```python
from build123d import *

# Parameters (mm, degrees)
RECESSII_CUT_EXTRUDE11_DEPTH = 2.0574
DRAFT2_ANGLE                 = 20
LPATTERN1_COUNT              = 9
LPATTERN1_PITCH              = 1.27


with BuildPart() as part:
    # Sketch1 → base-Revolve (revolve)
    with BuildSketch(Plane.XY, mode=Mode.PRIVATE) as base_revolve_sk:
        with BuildLine():
            Line((0, 0), (0, 2.2606))
            ThreePointArc((0, 2.2606), (0.342216437, 3.086783563), (1.1684, 3.429))
            Line((1.1684, 3.429), (2.0828, 3.429))
            Line((2.0828, 3.429), (2.0828, 1.7526))
            Line((2.0828, 1.7526), (14.7828, 1.7526))
            Line((14.7828, 1.7526), (14.7828, 0))
            Line((14.7828, 0), (0, 0))
        make_face()
    revolve(base_revolve_sk.sketch.rotate(Axis((0, 0, 0), (1, 0, 0)), 90), axis=Axis((0, 0, 0), (1, 0, 0)))

    # Sketch3 → recessII_Cut-Extrude11 (cut)
    with BuildSketch(Plane(origin=(0, 0, 0), x_dir=(0, 0, -1), z_dir=(1, 0, 0))):
        Polygon((0.4699, 2.1463), (-0.4699, 2.1463), (-0.4699, 0.4699), (-2.1463, 0.4699), (-2.1463, -0.4699), (-0.4699, -0.4699), (-0.4699, -2.1463), (0.4699, -2.1463), (0.4699, -0.4699), (2.1463, -0.4699), (2.1463, 0.4699), (0.4699, 0.4699), align=None)
    extrude(amount=RECESSII_CUT_EXTRUDE11_DEPTH, mode=Mode.SUBTRACT)

    # Draft2
    draft2_faces = [part.faces().sort_by_distance(p)[0] for p in [
        (1.0287, 0, -2.1463),
        (1.0287, -2.1463, 0),
        (1.0287, 0, 2.1463),
        (1.0287, 2.1463, 0),
    ]]
    draft(draft2_faces, Plane(origin=(0, 0, 0), x_dir=(0, 0, -1), z_dir=(-1, 0, 0)), DRAFT2_ANGLE)

    # thd_Sketch7 → thd_Cut-Revolve2 (revolve, cut)
    with BuildSketch(Plane.XY, mode=Mode.PRIVATE) as thd_cut_revolve2_sk:
        Polygon((3.3528, 1.7526), (3.602099846, 1.3208), (4.373500154, 1.3208), (4.6228, 1.7526), align=None)
    thd_cut_revolve2 = revolve(thd_cut_revolve2_sk.sketch.rotate(Axis((0, 0, 0), (1, 0, 0)), 90), axis=Axis((0, 0, 0), (1, 0, 0)), mode=Mode.SUBTRACT)

    # LPattern1: thd_Cut-Revolve2 ×9
    with Locations(*[(i * LPATTERN1_PITCH, 0, 0) for i in range(1, LPATTERN1_COUNT)]):
        add(thd_cut_revolve2, mode=Mode.SUBTRACT)

    # Sketch14 → point_Cut-Revolve3 (revolve, cut)
    with BuildSketch(Plane.XY, mode=Mode.PRIVATE) as point_cut_revolve3_sk:
        Polygon((14.7828, 0), (11.024337171, 1.7526), (14.967254292, 1.7526), (14.967254292, 0), align=None)
    revolve(point_cut_revolve3_sk.sketch.rotate(Axis((0, 0, 0), (1, 0, 0)), 90), axis=Axis((0, 0, 0), (1, 0, 0)), mode=Mode.SUBTRACT)


solid = part.part
```
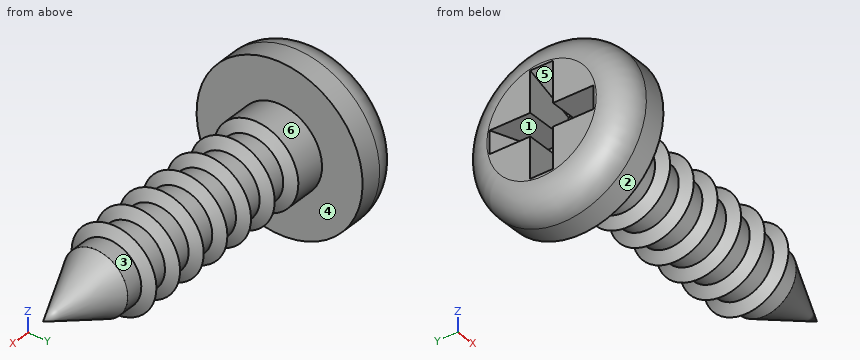
Check sheet for the modelled part. Datum: model origin and axes. Units: mm. Face numbers are marked on the shaded views. A direction names the side the tool comes from. Give positions to 0.01 mm unless a question says otherwise; leave off trailing zeros. Write each loop counter-clockwise with the first axis right and the second up, starting at its lowest first coordinate (ties: lowest second). Pieces come first, ordered by that corner, then holes.
Item 1: Cross-section at A-A (x = 3). Enter the section's corners in (y, z).
Item 2: Gauge pin test, flat ends, axial feed: pin 1 (4 mm diameter, centred on x = 8.5, z = -1, fed in from -Y); pin 2 (1.3 mm diameter, centred on x = 1.5, y = 1, fed in from -Z); pin 3 (0.8 mm diameter, centred on x = 1.5, z = -1.5, fed in from -Y). Record the tip position at first contact, or that the pin passes through.
Item 3: Access from +Z, -Z, +X, -X, +Y, -Y to the whole of each face (thin tool, end or side, straight path). Record for the marked faces 1, 2 and 3.
Item 4: Draft check along Z on the marked faces 4, 5 and 6. Enter one of: released by +Z, released by -Z, zero draft, split by the parting line, or undercut.
Item 5: Cross-section at B-B (x = 13.75). Enter the section's corners in (y, z).
Item 6: Scan lines: L1, parallel to X at y = -1.75, z = 0.75; L2, parallel to Z at x = 10, y = 0.5; L3, parallel to Y at x = 1, z = 2. Record each from-to range of solid material in increasing order.
Report:
1. outline: circle Ø3.51 at (0, 0)
2. pin 1: stops at y = -1.75
2. pin 2: stops at z = -3.41
2. pin 3: stops at y = -3.25
3. face 1: -X
3. face 2: +X, -X
3. face 3: +X
4. face 4: zero draft
4. face 5: undercut
4. face 6: split by the parting line
5. outline: circle Ø0.96 at (0, 0)
6. L1: x = 0 to 2.08
6. L2: z = -1.22 to 1.22
6. L3: y = -2.77 to 2.77
